```python
from build123d import *

# Parameters (mm, degrees)
F0_R      = 11
F1_DEPTH  = 3
F2_R      = 1
F3_R      = 9
F4_DEPTH  = 4
F5_R      = 4
F5_R_2    = 2.25
F6_DEPTH  = 9
F7_R      = 2
F8_DEPTH  = 1
F10_DEPTH = 3.6
F11_SIZE  = 0.5


with BuildPart() as f1:
    # F0 (on Right) → F1 (new body, symmetric)
    with BuildSketch(Plane.YZ):
        Circle(F0_R)
    extrude(amount=F1_DEPTH, both=True)

    # F2
    f2_edges = [f1.edges().sort_by_distance(p)[0] for p in [
        (-3, -11, 0),
        (3, -11, 0),
    ]]
    fillet(f2_edges, radius=F2_R)

    # F3 (on face) → F4 (cut)
    with BuildSketch(Plane(origin=(-3, 0, 0), x_dir=(0, -1, 0), z_dir=(-1, 0, 0))):
        Circle(F3_R)
    extrude(amount=-F4_DEPTH, mode=Mode.SUBTRACT)

    # F5 (on face) → F6 (join)
    with BuildSketch(Plane(origin=(1, 0, 0), x_dir=(0, -1, 0), z_dir=(-1, 0, 0))):
        Circle(F5_R)
        Circle(F5_R_2, mode=Mode.SUBTRACT)
    extrude(amount=F6_DEPTH)

    # F7 (on face) → F8 (join)
    with BuildSketch(Plane.YZ.offset(3)):
        Circle(F7_R)
    extrude(amount=F8_DEPTH)

    # F9 (on face) → F10 (join)
    with BuildSketch(Plane.YZ.offset(4)):
        Polygon((0.865, -0.499408), (0.865, 0.499408), (0, 0.998816), (-0.865, 0.499408), (-0.865, -0.499408), (0, -0.998816), align=None)
    extrude(amount=F10_DEPTH)

    # F11
    f11_edges = [f1.edges().sort_by_distance(p)[0] for p in [
        (-8, 4, 0),
    ]]
    chamfer(f11_edges, length=F11_SIZE)


solid = f1.part
```
Model file for the job. Use its own axes, mm. A direction names the side the tool comes from. Coordinates: 2 decimals unless noted, no trailing zeros. Order: outer loops, then holes, each group sorted by start corner. A loop starts at its lowest first (then second) coordinate and runs counter-clockwise, first axis right, second up. Notation, with made-up numbers: (-38, 64.25) -> (-18, 64.25) arc R4 ccw to (-18, 68.25) -> close; hole circle Ø7 at (-20, 43.5). An arc over 180 degrees is marked (long way). Answer as a JSON object with one key per item and string values. Group by question number.
1) Cut at A-A, the plane x = -0.5. Write the cut outline in (y, z).
2) Which spindle directions (+Z, -Z, +X, -X, +Y, -Y) get a long thin tool onto all of the face, cutting with end or side? Do faces 1 (the face through (5.775, 0.439, 0.746)), 2 (the face through (4, -0.5, -0.9)), 3 (the face through (6, -0.865, 0)). Say none if no direction does.
3) Pull direction Z, two halves, no side cores. Call faces 4 (the face through (-3.44, 0.29, 2.23)), 5 (the face through (5.77, -0.43, 0.75)), 6 (the face through (1, -4, -2)), 7 (the face through (-8, -0.7, -2.3)): +Z half, -Z half, draft (parallel to the pull), parting line (faces both ways), or undercut.
4) Flat gauge pins, fed straight in: pin 1 (0.5 mm diameter, centred on x = 6, z = 0, fed in from +Y) (3 decimals); pin 2 (3 mm diameter, centred on x = -1.5, y = 7, fed in from +Z); pin 3 (0.8 mm diameter, centred on x = 5.5, z = 0, fed in from -Y) (3 decimals); pin 4 (10 mm diameter, centred on y = -1.5, z = -4.5, fed in from -X). Where does each tip first touch, or does it go through?
5) Drill centre lines: L1, parallel to Z at x = -1.3, y = 0; L2, parallel to Z at x = -4.5, y = 0; L3, parallel to Z at x = -2, y = 3. Where is each one in solid material? Low to high.
Check values:
{
 "1": {"outline": "circle Ø22 at (0, 0); circle Ø8 at (0, 0); hole circle Ø18 at (0, 0); hole circle Ø4.5 at (0, 0)"},
 "2": {"face 1": "+Z, +X, +Y", "face 2": "+X", "face 3": "+Z, -Z, +X, -Y"},
 "3": {"face 4": "undercut", "face 5": "+Z half", "face 6": "undercut", "face 7": "draft"},
 "4": {"pin 1": "stops at y = 0.865", "pin 2": "stops at z = 9.53", "pin 3": "stops at y = -0.865", "pin 4": "stops at x = -8"},
 "5": {"L1": "z = -11 to -9, -4 to -2.25, 2.25 to 4, 9 to 11", "L2": "z = -4 to -2.25, 2.25 to 4", "L3": "z = -10.58 to -8.49, -2.65 to 2.65, 8.49 to 10.58"}
}
